from build123d import *

# Parameters (mm, degrees)
F0_R      = 152.4
F0_R_2    = 117.475
F1_DEPTH  = 25.4
F2_W      = 6.35
F2_H      = 9.525
F6_D      = 6.5278
F9_D      = 6.5278
F11_DEPTH = 3.175


with BuildPart() as f1:
    # F0 (on Front) → F1 (new body, symmetric)
    with BuildSketch(Plane.XZ):
        Circle(F0_R)
        Circle(F0_R_2, mode=Mode.SUBTRACT)
    extrude(amount=F1_DEPTH, both=True)

    # F2 (on Top) → F3 (revolve, cut)
    with BuildSketch(Plane.XY):
        with Locations((-149.225, 0)):
            Rectangle(F2_W, F2_H)
    revolve(axis=Axis((0, -5.8908760548, 0), (0, 1, 0)), mode=Mode.SUBTRACT)

    # F6 (through all)
    with Locations(Plane(origin=(0, 0, -152.4), x_dir=(1, 0, 0), z_dir=(0, 0, -1))):
        with Locations((0, 0)):
            Hole(F6_D / 2)

    # F9 (through all)
    with Locations(Plane.YZ.offset(152.4)):
        with Locations((0, 0)):
            Hole(F9_D / 2)

    # F10 (on face) → F11 (join)
    with BuildSketch(Plane.XZ.offset(25.4)):
        Polygon((31.75, 130.175), (-31.75, 130.175), (-31.75, 117.475), (-19.05, 104.775), (19.05, 104.775), (31.75, 117.475), align=None)
        Polygon((-130.175, 31.75), (-130.175, -31.75), (-117.475, -31.75), (-104.775, -19.05), (-104.775, 19.05), (-117.475, 31.75), align=None)
        Polygon((-31.75, -130.175), (31.75, -130.175), (31.75, -117.475), (19.05, -104.775), (-19.05, -104.775), (-31.75, -117.475), align=None)
        Polygon((130.175, -31.75), (130.175, 31.75), (117.475, 31.75), (104.775, 19.05), (104.775, -19.05), (117.475, -31.75), align=None)
    extrude(amount=F11_DEPTH)


solid = f1.part
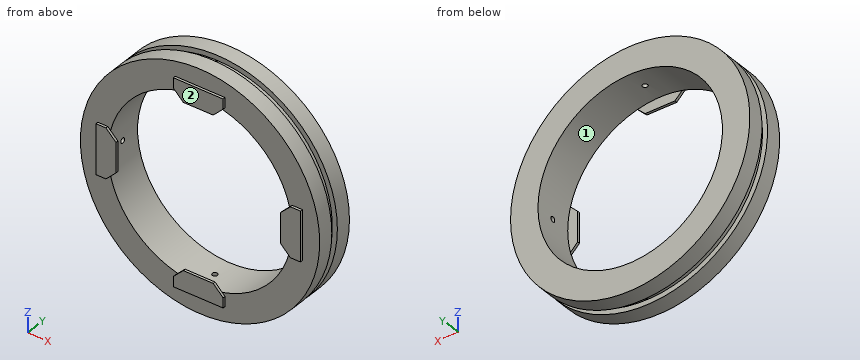
Read the model definition and answer for the solid it produces. Units are mm, in the model's axes. Face numbers are marked on the shaded views. Round coordinates to 2 decimals unless told otherwise and drop trailing zeros. Write each loop counter-clockwise with the first axis right and the second up, starting at its lowest first coordinate (ties: lowest second). Pieces come first, ordered by that corner, then holes. Notation, with made-up numbers: (-22.75, 16.5) - (13.25, 16.5) arc R22 ccw to (13.25, 48.5) - close; hole circle Ø7 at (30.25, 64.25). An arc over 180 degrees is marked (long way). Use a Markdown table: item, result.
(1) Straight lines are drawn through the part: line 1 along Y through (x, z) = (124.5, 0) (3 decimals); line 2 along Z through (x, y) = (0, 7) (3 decimals); line 3 along X through (y, z) = (-4.5, 0) (3 decimals). For each, find the intervals that lie inside material, in ascending order. Write a range as [from, to].
Reported:
| item | result |
|---|---|
| line 1 | [-28.575, -3.264], [3.264, 25.4] |
| line 2 | [-152.4, -117.475], [117.475, 152.4] |
| line 3 | [-146.05, -117.475], [117.475, 146.05] |
(2) The mould has two halves that part along Z. Classify the marked faces 1 and 2: released by +Z, released by -Z, zero draft, split by the parting line, or undercut.
Reported:
| item | result |
|---|---|
| face 1 | undercut |
| face 2 | zero draft |
(3) The part is cut by section A-A (z = -46). Write down the section's boundary in (x, y).
Reported:
| item | result |
|---|---|
| outline | (-145.29, -25.4) - (-108.09, -25.4) - (-108.09, 25.4) - (-145.29, 25.4) - (-145.29, 4.76) - (-138.62, 4.76) - (-138.62, -4.76) - (-145.29, -4.76) - close; (108.09, -25.4) - (145.29, -25.4) - (145.29, -4.76) - (138.62, -4.76) - (138.62, 4.76) - (145.29, 4.76) - (145.29, 25.4) - (108.09, 25.4) - close |
(4) Each of these flat-tipped pins is pushed along its axis until it touches: pin 1 Ø2.5 at (y, z) = (-26.5, -3.5) entering from -X; pin 2 Ø8 at (y, z) = (10.5, 92.5) entering from -X; pin 3 Ø2.5 at (x, y) = (-124, -27) entering from -Z; pin 4 Ø4 at (y, z) = (0, 0) entering from +X. Where does it stop, or does it pass through?
Reported:
| item | result |
|---|---|
| pin 1 | x = -152.37 |
| pin 2 | x = -124.07 |
| pin 3 | z = -31.75 |
| pin 4 | through |
(5) The part is cut by section B-B (x = -90). Write down the section's boundary in (y, z), then the cut area to 3 significant figures.
Reported:
| item | result |
|---|---|
| outline | (-25.4, -122.99) - (-4.76, -122.99) - (-4.76, -115.02) - (4.76, -115.02) - (4.76, -122.99) - (25.4, -122.99) - (25.4, -75.5) - (-25.4, -75.5) - close; (-25.4, 75.5) - (25.4, 75.5) - (25.4, 122.99) - (4.76, 122.99) - (4.76, 115.02) - (-4.76, 115.02) - (-4.76, 122.99) - (-25.4, 122.99) - close |
| area | 4,670 mm2 |
(6) The part is cut by section D-D (y = 10). Write down the section's boundary in (x, z) (3 decimals).
Reported:
| item | result |
|---|---|
| outline | circle Ø304.8 at (0, 0); hole circle Ø234.95 at (0, 0) |
(7) The part is cut by section C-C (x = 109). Write down the section's boundary in (y, z) (1 decimal).
Reported:
| item | result |
|---|---|
| outline | (-28.6, -23.3) - (-25.4, -23.3) - (-25.4, 23.3) - (-28.6, 23.3) - close; (-25.4, -106.5) - (-4.8, -106.5) - (-4.8, -97.2) - (4.8, -97.2) - (4.8, -106.5) - (25.4, -106.5) - (25.4, -43.8) - (-25.4, -43.8) - close; (-25.4, 43.8) - (25.4, 43.8) - (25.4, 106.5) - (4.8, 106.5) - (4.8, 97.2) - (-4.8, 97.2) - (-4.8, 106.5) - (-25.4, 106.5) - close |
